Build history of the part. All positions in model axes, mm. Give positions to 0.01 mm unless a question says otherwise; leave off trailing zeros. Order: outer loops, then holes, each group sorted by start corner. A loop starts at its lowest first (then second) coordinate and runs counter-clockwise, first axis right, second up. Notation, with made-up numbers: M 23.25,40 L 55.25,40 A14 ccw 55.25,46 Z; hole C 78.5,-17 d5. An arc over 180 degrees is marked long. Answer as CSV lines item,"result".
from build123d import *

# Parameters (mm, degrees)
SKETCH1_W           = 300
SKETCH1_H           = 100
BOSS_EXTRUDE1_DEPTH = 50
FILLET1_R           = 45


with BuildPart() as part:
    # Sketch1 → Boss-Extrude1 (new, symmetric)
    with BuildSketch(Plane.XY):
        Rectangle(SKETCH1_W, SKETCH1_H)
    extrude(amount=BOSS_EXTRUDE1_DEPTH, both=True)

    # Fillet1
    fillet1_edges = [part.edges().sort_by_distance(p)[0] for p in [
        (150, 0, 50),
        (0, 50, 50),
        (-150, 0, 50),
        (0, 50, -50),
        (150, 0, -50),
        (0, -50, -50),
        (-150, 0, -50),
        (-150, 50, 0),
        (150, 50, 0),
        (150, -50, 0),
        (-150, -50, 0),
        (0, -50, 50),
    ]]
    fillet(fillet1_edges, radius=FILLET1_R)


solid = part.part
Item 1: Pull direction Y, two halves, no side cores. Call faces 1 (the cylindrical face through (-137.168, -36.468, 0.07)), 2 (the cylindrical face through (137.168, 36.468, -0.07)), 3 (the flat face through (150, 0, 0)): released by +Y, released by -Y, zero draft, split by the parting line, or undercut.
Geometry says:
face 1,"released by -Y"
face 2,"released by +Y"
face 3,"zero draft"
Item 2: Drop flat-ended pins along their axis: pin 1 (6 mm diameter, centred on x = -73.5, z = 33.5, fed in from +Y); pin 2 (3 mm diameter, centred on y = 34.5, z = 2.5, fed in from -X); pin 3 (2 mm diameter, centred on x = -89, y = -14.5, fed in from +Z). Give the stop position or say it passes through.
Geometry says:
pin 1,"stops at y = 42.08"
pin 2,"stops at x = -140.23"
pin 3,"stops at z = 49.19"
Item 3: Band-saw the part on A-A (x = 78). Give the cut face in (y, z), and give its area (3 significant figures).
Geometry says:
outline,"M -50,-5 A45 ccw -5,-50 L 5,-50 A45 ccw 50,-5 L 50,5 A45 ccw 5,50 L -5,50 A45 ccw -50,5 Z"
area,"8,260 mm2"
Item 4: Probe line 1 along Y through (x, z) = (5, -5.5); line 2 along X through (y, z) = (-14.5, 17); line 3 along Z through (x, y) = (58, -17.5). List the from-to ranges inside material, lowest first. Write a range as from..to.
Geometry says:
line 1,"y = -50..50"
line 2,"x = -147.32..147.32"
line 3,"z = -48.23..48.23"
Item 5: Band-saw the part on B-B (y = 1). Give the cut face in (x, z), and give its area (3 significant figures).
Geometry says:
outline,"M -150,-5 A45 ccw -105,-50 L 105,-50 A45 ccw 150,-5 L 150,5 A45 ccw 105,50 L -105,50 A45 ccw -150,5 Z"
area,"28,300 mm2"
